```python
from build123d import *

# Parameters (mm, degrees)
SKETCH1_W               = 88.9
SKETCH1_H               = 25.4
BOSS_EXTRUDE1_DEPTH     = 4
MIRROR3_COPY_1_SKETCH_W = 88.9
MIRROR3_COPY_1_SKETCH_H = 25.4
MIRROR3_COPY_1_DEPTH    = 4


with BuildPart() as part:
    # Sketch1 → Boss-Extrude1 (new body)
    with BuildSketch(Plane(origin=(0, 0, 0), x_dir=(1, 0, 0), z_dir=(0, 1, 0))):
        Rectangle(SKETCH1_W, SKETCH1_H)
        Polygon((-44.45, 34.29), (-44.45, 12.7), (-31.75, 12.7), (-31.75, 34.29), (-38.1, 34.29), align=None)
    boss_extrude1 = extrude(amount=BOSS_EXTRUDE1_DEPTH)

    # Mirror1: Boss-Extrude1 across plane
    add(boss_extrude1.mirror(Plane.ZY))

    # Mirror2: Boss-Extrude1 across plane
    add(boss_extrude1.mirror(Plane.XY))

    # Mirror3: Boss-Extrude1 across plane
    add(boss_extrude1.mirror(Plane.ZY))

    # Mirror3 copy 1 sketch → Mirror3 copy 1 (add)
    with BuildSketch(Plane(origin=(0, 0, 0), x_dir=(-1, 0, 0), z_dir=(0, 1, 0))):
        Rectangle(MIRROR3_COPY_1_SKETCH_W, MIRROR3_COPY_1_SKETCH_H)
        Polygon((-44.45, 34.29), (-44.45, 12.7), (-31.75, 12.7), (-31.75, 34.29), (-38.1, 34.29), align=None)
    extrude(amount=MIRROR3_COPY_1_DEPTH)


solid = part.part
```
Model file for the job. Use its own axes, mm. A direction names the side the tool comes from. Coordinates: 2 decimals unless noted, no trailing zeros. Loops run counter-clockwise (first coordinate to the right, second up) from the corner with the lowest first, then second, coordinate; pieces in that order, holes last. Notation, with made-up numbers: (75.25, 2) -> (134.25, 2) arc R24 ccw to (134.25, 33) -> close; hole circle Ø9 at (17, 56). An arc over 180 degrees is marked (long way). Answer as a JSON object with one key per item and string values.
Q1. Pull direction X, two halves, no side cores. Call faces 4 (the flat face through (-44.45, 2, 0)), 5 (the flat face through (0, 2, -12.7)), 6 (the flat face through (-1, 4, 0)), 7 (the flat face through (44.45, 2, 0)): released by +X, released by -X, zero draft, split by the parting line, or undercut.
Report:
{"face 4": "released by -X", "face 5": "undercut", "face 6": "zero draft", "face 7": "released by +X"}
Q2. Cut at C-C (x = 10). List the corners of the cut face in (y, z), and give its area (3 significant figures).
Report:
{"outline": "(0, -12.7) -> (4, -12.7) -> (4, 12.7) -> (0, 12.7) -> close", "area": "102 mm2"}
Q3. Probe probe 1 along X at (y, z) = (2.45, -25.5); probe 2 along Z at (x, y) = (-7, 0.75). List the from-to ranges inside material, lowest first.
Report:
{"probe 1": "x = -44.45 to -31.75, 31.75 to 44.45", "probe 2": "z = -12.7 to 12.7"}
Q4. Cut at A-A (z = -14.5). List the corners of the cut face in (x, y).
Report:
{"outline": "(-44.45, 0) -> (-31.75, 0) -> (-31.75, 4) -> (-44.45, 4) -> close; (31.75, 0) -> (44.45, 0) -> (44.45, 4) -> (31.75, 4) -> close"}
Q5. Cut at B-B (y = 0.65). List the corners of the cut face in (x, z), and give its area (3 significant figures).
Report:
{"outline": "(-44.45, -34.29) -> (-31.75, -34.29) -> (-31.75, -12.7) -> (31.75, -12.7) -> (31.75, -34.29) -> (44.45, -34.29) -> (44.45, 34.29) -> (31.75, 34.29) -> (31.75, 12.7) -> (-31.75, 12.7) -> (-31.75, 34.29) -> (-44.45, 34.29) -> close", "area": "3,350 mm2"}
Q6. 3-axis set-ups, long thin cutter, end or side, ignore diameter. For faces 1 (the flat face through (-31.75, 2, -23)), 2 (the flat face through (-38, 2, -34.29)), 3 (the flat face through (-31.75, 2, 23)): which of +Z, -Z, +X, -X, +Y, -Y reach the whole face in a straight line?
Report:
{"face 1": "-Z, +Y, -Y", "face 2": "-Z, +X, -X, +Y, -Y", "face 3": "+Z, +Y, -Y"}
Q7. Flat gauge pins, fed straight in: P1, Ø2, axis at x = 15.5, y = 2, coming from the +Z side; P2, Ø1.2, axis at x = -13, y = 2, coming from the -Z side. Where does each tip first touch, or does it go through?
Report:
{"P1": "stops at z = 12.7", "P2": "stops at z = -12.7"}
